The listing builds one solid part. Answer for the finished solid, in the listing's coordinates (mm). A direction names the side the tool comes from. Round coordinates to 2 decimals unless told otherwise and drop trailing zeros. Order: outer loops, then holes, each group sorted by start corner. A loop starts at its lowest first (then second) coordinate and runs counter-clockwise, first axis right, second up. Notation, with made-up numbers: (-2.5, 63) - (5.5, 63) arc R22 cw to (5.5, 75) - close; hole circle Ø7 at (-1.75, -35). An arc over 180 degrees is marked (long way). One line per item, written item: value. Start each with the question number.
1. Flat-ended cylindrical pins translate along their axes: P1, Ø10.5, axis at x = 23, y = 7.5, coming from the +Z side; P2, Ø2, axis at y = -16, z = 7.5, coming from the +X side; P3, Ø2.5, axis at x = 1, z = 11, coming from the -Y side. Find the tip coordinate at first contact, or state that the pin passes through.
2. For a pull along Y with two mould halves and no side action, classify faces 4 (the cylindrical face through (-17.496, 0.385, 1.972)), 5 (the flat face through (-2, -15, 9)), 6 (the flat face through (18, 0, 2)), 7 (the flat face through (19, 17.5, 2)) as released by +Y, released by -Y, zero draft, split by the parting line, or undercut.
3. Straight lines are drawn through the part: line 1 (Y direction, x = 27, z = 10.4); line 2 (Y direction, x = 26, z = 11.25); line 3 (X direction, y = 7, z = 3.25). For each, find the intervals that lie inside material, in ascending order.
4. Section B-B, the plane z = 6.5 is taken. Give the vertices of the cut face in (x, y), then the cut area to 3 significant figures.
5. Section D-D, the plane z = 2 is taken. Give the vertices of the cut face in (x, y).
6. Section C-C, the plane y = 2 is taken. Give the vertices of the cut face in (x, z).
7. A tool of negligible diameter and unlimited length cuts with its end or side. For faces 1 (the flat face through (33, -15, 9)), 2 (the flat face through (-9, 0, 2)), 3 (the cylindrical face through (27.668, -14.79, 10.842)), from which of +Z, -Z, +X, -X, +Y, -Y can it reach the whole face along a straight path? Write none if from no direction.
8. Section A-A, the plane x = 17 is taken. Give the vertices of the cut face in (y, z), then the cut area to 3 significant figures.
from build123d import *

# Parameters (mm, degrees)
PAD_DEPTH       = 4
SKETCH001_W     = 8
SKETCH001_H     = 4
PAD001_DEPTH    = 9.8
SKETCH002_R     = 7.6
POCKET_DEPTH    = 5
SKETCH003_R     = 0.7
POCKET001_DEPTH = 6
SKETCH004_W     = 4
SKETCH004_H     = 18
POCKET002_DEPTH = 5


with BuildPart() as part:
    # Sketch → Pad (new body)
    with BuildSketch(Plane.XY):
        with BuildLine():
            ThreePointArc((-3e-06, 17.5), (-17.5, -1.8e-05), (3.3e-05, -17.5))
            Line((3.3e-05, -17.5), (38, -17.5))
            Line((38, 17.500005), (38, -17.5))
            Line((-3e-06, 17.5), (38, 17.500005))
        make_face()
    extrude(amount=PAD_DEPTH)

    # Sketch001 → Pad001 (new body)
    with BuildSketch(Plane.XY.offset(4)):
        with Locations((2, 15)):
            Rectangle(SKETCH001_W, SKETCH001_H)
        with Locations((2, -15)):
            Rectangle(SKETCH001_W, SKETCH001_H)
        with Locations((29, 15)):
            Rectangle(SKETCH001_W, SKETCH001_H)
        with Locations((29, -15)):
            Rectangle(SKETCH001_W, SKETCH001_H)
    extrude(amount=PAD001_DEPTH)

    # Sketch002 → Pocket (cut)
    with BuildSketch(Plane.XY.offset(4)):
        with Locations((2, 0)):
            Circle(SKETCH002_R)
        with Locations((29, 0)):
            Circle(SKETCH002_R)
    extrude(amount=-POCKET_DEPTH, mode=Mode.SUBTRACT)

    # Sketch003 → Pocket001 (cut)
    with BuildSketch(Plane.XY.offset(13.8)):
        with Locations((0, 15)):
            Circle(SKETCH003_R)
        with Locations((27, 15)):
            Circle(SKETCH003_R)
        with Locations((27, -15)):
            Circle(SKETCH003_R)
        with Locations((0, -15)):
            Circle(SKETCH003_R)
    extrude(amount=-POCKET001_DEPTH, mode=Mode.SUBTRACT)

    # Sketch004 → Pocket002 (cut)
    with BuildSketch(Plane.XY.offset(4)):
        with Locations((-11, 0)):
            Rectangle(SKETCH004_W, SKETCH004_H)
        with Locations((16, 0)):
            Rectangle(SKETCH004_W, SKETCH004_H)
    extrude(amount=-POCKET002_DEPTH, mode=Mode.SUBTRACT)


solid = part.part
Answer list:
1. P1: stops at z = 4
1. P2: stops at x = 33
1. P3: stops at y = -17
2. face 4: split by the parting line
2. face 5: zero draft
2. face 6: undercut
2. face 7: released by +Y
3. line 1: y = -17 to -15.7, -14.3 to -13, 13 to 14.3, 15.7 to 17
3. line 2: y = -17 to -13, 13 to 17
3. line 3: x = -16.04 to -13, -9 to -0.96, 4.96 to 14, 18 to 26.04, 31.96 to 38
4. outline: (-2, -17) - (6, -17) - (6, -13) - (-2, -13) - close; (-2, 13) - (6, 13) - (6, 17) - (-2, 17) - close; (25, -17) - (33, -17) - (33, -13) - (25, -13) - close; (25, 13) - (33, 13) - (33, 17) - (25, 17) - close
4. area: 128 mm²
5. outline: (0, -17.5) - (38, -17.5) - (38, 17.5) - (0, 17.5) arc R17.5 ccw to start; hole (-13, -9) - (-9, -9) - (-9, 9) - (-13, 9) - close; hole circle Ø15.2 at (2, 0); hole (14, -9) - (18, -9) - (18, 9) - (14, 9) - close; hole circle Ø15.2 at (29, 0)
6. outline: (-17.39, 0) - (-13, 0) - (-13, 4) - (-17.39, 4) - close; (-9, 0) - (-5.33, 0) - (-5.33, 4) - (-9, 4) - close; (9.33, 0) - (14, 0) - (14, 4) - (9.33, 4) - close; (18, 0) - (21.67, 0) - (21.67, 4) - (18, 4) - close; (36.33, 0) - (38, 0) - (38, 4) - (36.33, 4) - close
7. face 1: +Z, +X, +Y, -Y
7. face 2: +Z, -Z
7. face 3: +Z
8. outline: (-17.5, 0) - (-9, 0) - (-9, 4) - (-17.5, 4) - close; (9, 0) - (17.5, 0) - (17.5, 4) - (9, 4) - close
8. area: 68.0 mm²
